The model under review builds one solid part; all positions refer to its coordinate system, in mm. Face numbers are marked on the shaded views. A direction names the side the tool comes from. Coordinates: 2 decimals unless noted, no trailing zeros. Loops run counter-clockwise (first coordinate to the right, second up) from the corner with the lowest first, then second, coordinate; pieces in that order, holes last. Notation, with made-up numbers: M -7,31.25 L 33,31.25 A16 ccw 33,58.25 Z; hole C 6.5,0.25 d6. An arc over 180 degrees is marked long. One line per item, written item: value.
```python
from build123d import *

# Parameters (mm, degrees)
SKETCH1_R               = 25.4
BOSS_EXTRUDE1_DEPTH     = 73.025
SKETCH2_R               = 14.2875
CUT_EXTRUDE1_DEPTH      = 6.35
CUT_EXTRUDE2_START      = -6.35
SKETCH3_R               = 14.2875
CUT_EXTRUDE2_DEPTH      = 6.35
CUT_EXTRUDE3_DEPTH      = 76.735563806
CUT_EXTRUDE3_DEPTH_BACK = 76.735563806
SKETCH4_R               = 8.763
SKETCH5_R               = 25.4
SKETCH5_R_2             = 16.51
CUT_EXTRUDE5_DEPTH      = 17.78
FILLET8_R               = 1.5875


with BuildPart() as part:
    # Sketch1 → Boss-Extrude1 (new body)
    with BuildSketch(Plane(origin=(0, 0, 0), x_dir=(1, 0, 0), z_dir=(0, 1, 0))):
        with Locations(Location((0, 0, 0), (0, 0, 270))):
            Circle(SKETCH1_R)
    extrude(amount=BOSS_EXTRUDE1_DEPTH)

    # Sketch2 → Cut-Extrude1 (cut)
    with BuildSketch(Plane(origin=(0, 73.025, 0), x_dir=(1, 0, 0), z_dir=(0, 1, 0))):
        with Locations(Location((0, 0, 0), (0, 0, 270))):
            Circle(SKETCH2_R)
    extrude(amount=-CUT_EXTRUDE1_DEPTH, mode=Mode.SUBTRACT)

    # Sketch3 → Cut-Extrude2 (cut)
    with BuildSketch(Plane.XZ.offset(CUT_EXTRUDE2_START)):
        with Locations(Location((0, 0, 0), (0, 0, 90))):
            Circle(SKETCH3_R)
    extrude(amount=CUT_EXTRUDE2_DEPTH, mode=Mode.SUBTRACT)

    # Sketch4 → Cut-Extrude3 (cut, two sides: drawn at the far end of the back side and taken through both)
    with BuildSketch(Plane.XZ.offset(-6.35).offset(-CUT_EXTRUDE3_DEPTH_BACK)):
        with Locations(Location((0, 0, 0), (0, 0, 270))):
            Circle(SKETCH4_R)
    extrude(amount=CUT_EXTRUDE3_DEPTH + CUT_EXTRUDE3_DEPTH_BACK, mode=Mode.SUBTRACT)

    # Sketch5 → Cut-Extrude5 (cut)
    with BuildSketch(Plane(origin=(0, 0, 0), x_dir=(-1, 0, 0), z_dir=(0, -1, 0))):
        with Locations(Location((0, 0, 0), (0, 0, 90))):
            Circle(SKETCH5_R)
        with Locations(Location((0, 0, 0), (0, 0, 90))):
            Circle(SKETCH5_R_2, mode=Mode.SUBTRACT)
    extrude(amount=-CUT_EXTRUDE5_DEPTH, mode=Mode.SUBTRACT)

    # Sketch10 → Revolve3 (revolve)
    with BuildSketch(Plane.XY, mode=Mode.PRIVATE) as revolve3_sk:
        with BuildLine():
            Line((-25.4, 17.78), (-16.51, 17.78))
            Line((-16.51, 17.78), (-16.51, 0))
            ThreePointArc((-16.51, 0), (-18.85635568, 9.93932216), (-25.4, 17.78))
        make_face()
    revolve(revolve3_sk.sketch.rotate(Axis((0, 0, 0), (0, -1, 0)), 90), axis=Axis((0, 0, 0), (0, -1, 0)))

    # Fillet8
    fillet8_edges = [part.edges().sort_by_distance(p)[0] for p in [
        (25.4, 17.78, 0),
        (0, 0, 16.51),
        (0, 73.025, -25.4),
    ]]
    fillet(fillet8_edges, radius=FILLET8_R)


solid = part.part
```
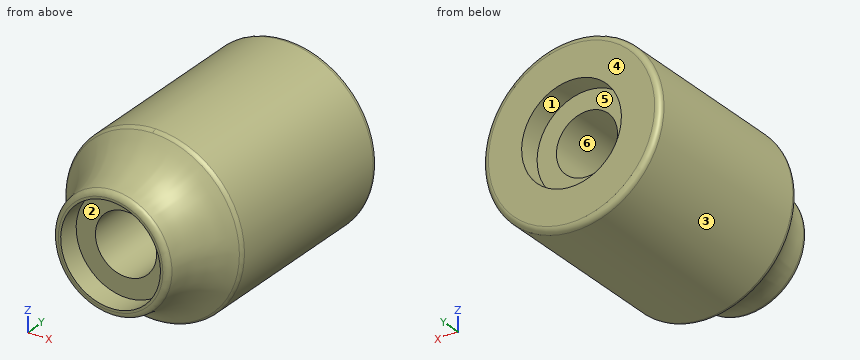
(1) Draft analysis for pull direction Z (two halves, no side actions). For the marked faces 3, 4, 5 and 6, state which applies: pulls with the +Z half, pulls with the -Z half, needs draft (parallel to the pull), parting line crosses it, or undercut.
Checks:
face 3: parting line crosses it
face 4: needs draft
face 5: undercut
face 6: undercut
(2) To check wall thickness, follow L1, parallel to X at y = 1.5, z = 0; L2, parallel to X at y = 20.5, z = -0.5; L3, parallel to Z at x = 0, y = 38. State the ranges of each line that lie inside material, in increasing order. Write a range as [from, to].
Checks:
L1: [-16.56, -14.29], [14.29, 16.56]
L2: [-25.4, -8.75], [8.75, 25.4]
L3: [-25.4, -8.76], [8.76, 25.4]
(3) Tool access review of the marked faces 1 and 2: name each direction out of +Z, -Z, +X, -X, +Y, -Y from which nothing blocks a thin tool from reaching the whole face with its end or side.
Checks:
face 1: +Y
face 2: -Y
(4) Add section A-A on y = 36. State the section outline as (x, z) points.
Checks:
outline: C 0,0 d50.8; hole C 0,0 d17.53
(5) Insertion check: pin 1 Ø2 at (x, z) = (-15.5, -2.5) entering from -Y; pin 2 Ø2 at (x, y) = (-9, 47.5) entering from -Z; pin 3 Ø1 at (x, z) = (7.5, 1.5) entering from +Y; pin 4 Ø23 at (x, z) = (0, 0) entering from -Y. Each pin has a flat end and moves straight along its axis. Give the tip position at first contact, or say it passes through.
Checks:
pin 1: y = 0
pin 2: z = -24.11
pin 3: through
pin 4: y = 6.35
